Here's how the part is built. I have some questions about the finished solid (model axes, mm). A direction names the side the tool comes from. Round coordinates to 2 decimals unless told otherwise and drop trailing zeros. Loops run counter-clockwise (first coordinate to the right, second up) from the corner with the lowest first, then second, coordinate; pieces in that order, holes last. Notation, with made-up numbers: (45.25, 56.5) - (78.25, 56.5) arc R26 ccw to (78.25, 71.5) - close; hole circle Ø3 at (1.5, 32.5). An arc over 180 degrees is marked (long way). Answer as a JSON object with one key per item and string values. Group by question number.
1) Will these pins go through, and if not, where does the flat tip stop? P1, Ø1.5, axis at x = 2, y = 5.5, coming from the -Z side; P2, Ø8, axis at y = 2.5, z = -6, coming from the +X side; P3, Ø5, axis at x = 0, y = 13.5, coming from the -Z side.
2) I want a section at B-B, the plane x = 0. Please give me the cut outline in (y, z), then the cut area to 3 significant figures.
3) I want a section at A-A, the plane z = 0. Please give me the cut outline in (x, y).
4) If I drill on line 1 along Y through (x, z) = (-3.55, 0); line 2 along Y through (x, z) = (-6.5, 5.75); line 3 along X through (y, z) = (12, 0), over which ranges is the centre line in solid material (lowest first)? Write a range as [from, to].
5) I want a section at D-D, the plane x = 2. Please give me the cut outline in (y, z).
6) Which directions (+Z, -Z, +X, -X, +Y, -Y) give clear straight access to the entire face, cutting with the end or side of a thin tool? Please do faces 4 (the face through (2.11, 8.87, 1.34)), 5 (the face through (-3.482, 2.536, 0.325)), 6 (the face through (4.88, 3.94, 1.08)), 7 (the face through (4, 16.5, -4)).
7) I want a section at C-C, the plane y = 9.75. Please give me the cut outline in (x, z), then the cut area to 3 significant figures.
8) If we mould it in two halves opening along Y, with no side actions, what happens to faces 1 (the face through (2, 0, -2)), 2 (the face through (-1.532, 12.698, -4.864)), 3 (the face through (-6.083, 8.493, 6.633))? For each: pulls with the +Y half, pulls with the -Y half, needs draft (parallel to the pull), parting line crosses it, or undercut.
from build123d import *

# Parameters (mm, degrees)
SKETCH3_R               = 2.5
CUT_EXTRUDE2_DEPTH      = 22.639085008
CUT_EXTRUDE3_REACH      = 23.639
CUT_EXTRUDE3_END_RADIUS = 5
SKETCH4_R               = 1.5


with BuildPart() as part:
    # Sketch1 → Revolve1 (revolve)
    with BuildSketch(Plane.XY, mode=Mode.PRIVATE) as revolve1_sk:
        Polygon((0, 0), (0, 17.5), (9, 17.5), (9, 16.5), (5.1, 16.5), (5.1, 9), (9, 9), (9, 8), (5, 8), (5, 0), align=None)
    revolve(revolve1_sk.sketch.rotate(Axis((0, 0, 0), (0, 1, 0)), 90), axis=Axis((0, 0, 0), (0, 1, 0)))

    # Sketch3 → Cut-Extrude2 (cut, through all)
    with BuildSketch(Plane(origin=(0, 17.5, 0), x_dir=(1, 0, 0), z_dir=(0, 1, 0))):
        with Locations(Location((0, 0, 0), (0, 0, 270))):
            Circle(SKETCH3_R)
    extrude(amount=-CUT_EXTRUDE2_DEPTH, mode=Mode.SUBTRACT)

    # Cut-Extrude3: up to this cylinder (the profile starts inside it)
    cut_extrude3_end = Plane(origin=(0, 4, 0), z_dir=(0, -1, 0)) * Cylinder(CUT_EXTRUDE3_END_RADIUS, 58.278, mode=Mode.PRIVATE)
    # Sketch4 → Cut-Extrude3 (cut, up to the surface)
    with BuildSketch(Plane(origin=(0, 0, 0), x_dir=(0, 0, -1), z_dir=(1, 0, 0)), mode=Mode.PRIVATE) as cut_extrude3_sk1:
        with Locations((0, 4)):
            Circle(SKETCH4_R)
    cut_extrude3_tool1 = extrude(cut_extrude3_sk1.sketch, amount=-CUT_EXTRUDE3_REACH, mode=Mode.PRIVATE) & cut_extrude3_end
    add(cut_extrude3_tool1.solids().sort_by_distance((0, 4, 0))[0], mode=Mode.SUBTRACT)


solid = part.part
Outcome:
{
 "1": {"P1": "z = -4.84", "P2": "x = 4.58", "P3": "z = -5.1"},
 "2": {"outline": "(0, -5) - (8, -5) - (8, -9) - (9, -9) - (9, -5.1) - (16.5, -5.1) - (16.5, -9) - (17.5, -9) - (17.5, -2.5) - (0, -2.5) - close; (0, 2.5) - (17.5, 2.5) - (17.5, 9) - (16.5, 9) - (16.5, 5.1) - (9, 5.1) - (9, 9) - (8, 9) - (8, 5) - (0, 5) - close", "area": "105 mm^2"},
 "3": {"outline": "(-9, 8) - (-5, 8) - (-5, 5.5) - (-2.5, 5.5) - (-2.5, 17.5) - (-9, 17.5) - (-9, 16.5) - (-5.1, 16.5) - (-5.1, 9) - (-9, 9) - close; (-5, 0) - (-2.5, 0) - (-2.5, 2.5) - (-5, 2.5) - close; (2.5, 0) - (5, 0) - (5, 8) - (9, 8) - (9, 9) - (5.1, 9) - (5.1, 16.5) - (9, 16.5) - (9, 17.5) - (2.5, 17.5) - close"},
 "4": {"line 1": "[0, 2.5], [5.5, 17.5]", "line 2": "[8, 9], [16.5, 17.5]", "line 3": "[-5.1, -2.5], [2.5, 5.1]"},
 "5": {"outline": "(0, -4.58) - (8, -4.58) - (8, -8.77) - (9, -8.77) - (9, -4.69) - (16.5, -4.69) - (16.5, -8.77) - (17.5, -8.77) - (17.5, -1.5) - (0, -1.5) - close; (0, 1.5) - (17.5, 1.5) - (17.5, 8.77) - (16.5, 8.77) - (16.5, 4.69) - (9, 4.69) - (9, 8.77) - (8, 8.77) - (8, 4.58) - (0, 4.58) - close"},
 "6": {"face 4": "+Y, -Y", "face 5": "-X", "face 6": "-Y", "face 7": "none"},
 "7": {"outline": "circle Ø10.2 at (0, 0); hole circle Ø5 at (0, 0)", "area": "62.1 mm^2"},
 "8": {"face 1": "pulls with the -Y half", "face 2": "undercut", "face 3": "needs draft"}
}
